```python
from build123d import *

# Parameters (mm, degrees)
EXTRUDE_1_DEPTH     = 2.4
SKETCH_2_OUTSIDE_W  = 17.954
SKETCH_2_OUTSIDE_H  = 17.118
SKETCH_2_OUTSIDE_R  = 2.7
CUT_EXTRUDE_1_DEPTH = 4
CUT_EXTRUDE_1_DRAFT = -45
SKETCH_3_OUTSIDE_W  = 17.954
SKETCH_3_OUTSIDE_H  = 17.118
SKETCH_3_OUTSIDE_R  = 2.7
CUT_EXTRUDE_2_DEPTH = 4
CUT_EXTRUDE_2_DRAFT = -45
SKETCH_3_2_R        = 2.7
EXTRUDE_2_DEPTH     = 1.6
FILLET_1_R          = 0.2
SKETCH_4_R          = 1.5
CUT_EXTRUDE_3_DEPTH = 6.745433016


with BuildPart() as part:
    # Sketch 1 → Extrude 1 (new body)
    with BuildSketch(Plane.XY):
        Polygon((-1.558845727, 2.7), (1.558845727, 2.7), (3.117691454, 0), (1.558845727, -2.7), (-1.558845727, -2.7), (-3.117691454, 0), align=None)
    extrude(amount=EXTRUDE_1_DEPTH)


with BuildPart() as cut_extrude_1_tool:
    # Sketch 2 outside → Cut-Extrude 1 (with draft: the straight prism first)
    with BuildSketch(Plane(origin=(0, 0, 0), x_dir=(-1, 0, 0), z_dir=(0, 0, -1))):
        Rectangle(SKETCH_2_OUTSIDE_W, SKETCH_2_OUTSIDE_H)
        Circle(SKETCH_2_OUTSIDE_R, mode=Mode.SUBTRACT)
    extrude(amount=-CUT_EXTRUDE_1_DEPTH)
    # Cut-Extrude 1: the draft: its side faces are tilted about the plane it starts from
    cut_extrude_1_sides = [cut_extrude_1_tool.faces().sort_by_distance(p)[0] for p in [
        (0, -8.559, 2),
        (-8.977, 0, 2),
        (0, 8.559, 2),
        (8.977, 0, 2),
        (2.7, 0, 2),
    ]]
    draft(cut_extrude_1_sides, Plane(origin=(0, 0, 0), x_dir=(-1, 0, 0), z_dir=(0, 0, -1)), CUT_EXTRUDE_1_DRAFT)


with BuildPart() as part_1:
    add(part.part)

    # Cut-Extrude 1: cut by cut_extrude_1_tool
    add(cut_extrude_1_tool.part, mode=Mode.SUBTRACT)


with BuildPart() as cut_extrude_2_tool:
    # Sketch 3 outside → Cut-Extrude 2 (with draft: the straight prism first)
    with BuildSketch(Plane.XY.offset(2.4)):
        Rectangle(SKETCH_3_OUTSIDE_W, SKETCH_3_OUTSIDE_H)
        Circle(SKETCH_3_OUTSIDE_R, mode=Mode.SUBTRACT)
    extrude(amount=-CUT_EXTRUDE_2_DEPTH)
    # Cut-Extrude 2: the draft: its side faces are tilted about the plane it starts from
    cut_extrude_2_sides = [cut_extrude_2_tool.faces().sort_by_distance(p)[0] for p in [
        (0, -8.559, 0.4),
        (8.977, 0, 0.4),
        (0, 8.559, 0.4),
        (-8.977, 0, 0.4),
        (-2.7, 0, 0.4),
    ]]
    draft(cut_extrude_2_sides, Plane.XY.offset(2.4), CUT_EXTRUDE_2_DRAFT)


with BuildPart() as part_2:
    add(part_1.part)

    # Cut-Extrude 2: cut by cut_extrude_2_tool
    add(cut_extrude_2_tool.part, mode=Mode.SUBTRACT)

    # Sketch 3_2 → Extrude 2 (add)
    with BuildSketch(Plane.XY.offset(2.4)):
        with Locations(Location((0, 0, 0), (0, 0, 150))):
            Circle(SKETCH_3_2_R)
    extrude(amount=EXTRUDE_2_DEPTH)

    # Fillet 1
    fillet_1_edges = [part_2.edges().sort_by_distance(p)[0] for p in [
        (2.33826859, -1.35, 4),
    ]]
    fillet(fillet_1_edges, radius=FILLET_1_R)

    # Sketch 4 → Cut-Extrude 3 (cut, through all)
    with BuildSketch(Plane.XY.offset(4)):
        Circle(SKETCH_4_R)
    extrude(amount=-CUT_EXTRUDE_3_DEPTH, mode=Mode.SUBTRACT)


solid = part_2.part
```
Build history of the part. All positions in model axes, mm. A direction names the side the tool comes from. Round coordinates to 2 decimals unless told otherwise and drop trailing zeros. Order: outer loops, then holes, each group sorted by start corner. A loop starts at its lowest first (then second) coordinate and runs counter-clockwise, first axis right, second up. Notation, with made-up numbers: (-2.75, 63) - (3.25, 63) arc R24 cw to (3.25, 101) - close; hole circle Ø11 at (11.25, 21). An arc over 180 degrees is marked (long way). Use a Markdown table: item, result.
1) Saw through at A-A on z = 1.6. Write the cut outline in (x, y).
Recorded:
| item | result |
|---|---|
| outline | (-3.12, 0) - (-1.56, -2.7) - (1.56, -2.7) - (3.12, 0) - (1.56, 2.7) - (-1.56, 2.7) - close; hole circle Ø3 at (0, 0) |
2) Pull direction Y, two halves, no side cores. Call faces 3 (the face through (-1.2, -1.2, 0)), 4 (the face through (0, -2.7, 1)), 5 (the face through (-1.5, 0.07, 2.03)): pulls with the +Y half, pulls with the -Y half, needs draft (parallel to the pull), parting line crosses it, or undercut.
Recorded:
| item | result |
|---|---|
| face 3 | needs draft |
| face 4 | pulls with the -Y half |
| face 5 | undercut |
3) Wall check: L1, parallel to Y at x = 0, z = 2.3; L2, parallel to X at y = -0.4, z = 3.45; L3, parallel to X at y = 0.75, z = 3.75. Give the ranges that are in metal, low to high.
Recorded:
| item | result |
|---|---|
| L1 | y = -2.7 to -1.5, 1.5 to 2.7 |
| L2 | x = -2.67 to -1.45, 1.45 to 2.67 |
| L3 | x = -2.59 to -1.3, 1.3 to 2.59 |
4) Tool access for faces 1 (the face through (-2.636, 0.585, 3.09)), 2 (the face through (0, 2.7, 1)): list every direction of +Z, -Z, +X, -X, +Y, -Y with a clear straight run to the whole face (end or side of a thin tool).
Recorded:
| item | result |
|---|---|
| face 1 | +Z |
| face 2 | +Z, -Z, +X, -X, +Y |
5) Saw through at B-B on z = 3.15. Write the cut outline in (x, y), and give its area (3 significant figures).
Recorded:
| item | result |
|---|---|
| outline | circle Ø5.4 at (0, 0); hole circle Ø3 at (0, 0) |
| area | 15.8 mm² |
6) Flat gauge pins, fed straight in: pin 1 Ø2.5 at (x, y) = (0, 0) entering from +Z; pin 2 Ø1 at (x, z) = (2, 0.5) entering from +Y. Where does each tip first touch, or does it go through?
Recorded:
| item | result |
|---|---|
| pin 1 | passes through |
| pin 2 | stops at y = 2.7 |
